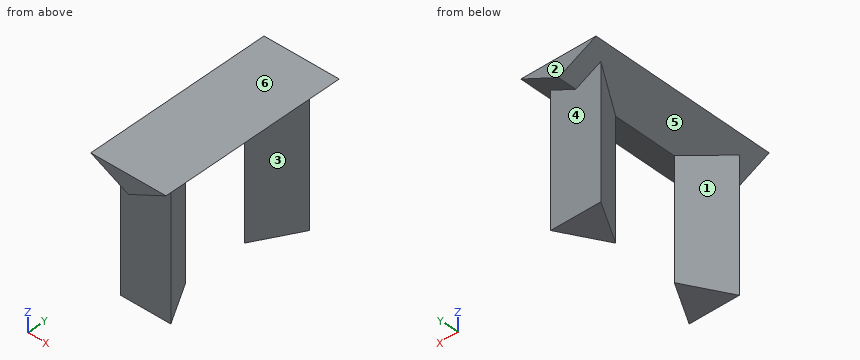
from build123d import *

# Parameters (mm, degrees)
F1_DEPTH = 150
F4_DEPTH = 110


with BuildPart() as f1:
    # F0 (on Front) → F1 (new body)
    with BuildSketch(Plane.XZ):
        Polygon((60, 0), (0, 0), (30, -15), align=None)
    extrude(amount=F1_DEPTH)

    # F3 (on offset) → F4 (join)
    with BuildSketch(Plane.XY.offset(-110)):
        Polygon((30, -100.3589838486), (10, -135), (50, -135), align=None)
        Polygon((30, -49.6410161514), (50, -15), (10, -15), align=None)
    extrude(amount=F4_DEPTH)


solid = f1.part
Can you work these out from the model? Positions are in its coordinate system, mm. Face numbers are marked on the shaded views. A direction names the side the tool comes from. Give positions to 0.01 mm unless a question says otherwise; leave off trailing zeros. Write each loop counter-clockwise with the first axis right and the second up, starting at its lowest first coordinate (ties: lowest second). Pieces come first, ordered by that corner, then holes. Notation, with made-up numbers: (36.25, 51.25) -> (64.25, 51.25) arc R27 ccw to (64.25, 76.25) -> close; hole circle Ø3 at (-35.5, 5.5). An arc over 180 degrees is marked (long way). Answer as a JSON object with one key per item and string values. Group by question number.
Item 1: I'm going to push flat-ended pins straight in: P1, Ø20, axis at x = 34.5, z = -35, coming from the -Y side; P2, Ø4, axis at x = 17, y = -106.5, coming from the -Z side; P3, Ø1, axis at x = 44, z = -73.5, coming from the +Y side. Where does each tip first touch, or does it pass through?
Item 2: Suppose I cut it at D-D (x = 46). Please give me the cut outline in (y, z).
Item 3: Please list where these lines run through material, in increasing order: line 1 (Y direction, x = 18, z = -18.5); line 2 (Y direction, x = 20, z = -44); line 3 (Z direction, x = 39, y = -79.5). Write a range as [from, to].
Item 4: Suppose I cut it at A-A (z = -95.5). Please give me the cut outline in (x, y).
Item 5: Suppose I cut it at C-C (y = -115). Please give me the cut outline in (x, z), plus the area to 3 significant figures.
Item 6: Suppose I cut it at B-B (x = 53). Please give me the cut outline in (y, z).
Item 7: For the marked faces 1, 2 and 3, which set-ups out of +Z, -Z, +X, -X, +Y, -Y let a thin tool reach every point of the face, with its end or its side?
Item 8: We'd pull the mould along Y, two halves only. Please class the marked faces 4, 5 and 6: +Y half, -Y half, draft (parallel to the pull), parting line (faces both ways), or undercut.
Findings:
{
 "1": {"P1": "stops at y = -135", "P2": "stops at z = -9.5", "P3": "stops at y = -15"},
 "2": {"outline": "(-150, -7) -> (-135, -7) -> (-135, -110) -> (-128.07, -110) -> (-128.07, -7) -> (-21.93, -7) -> (-21.93, -110) -> (-15, -110) -> (-15, -7) -> (0, -7) -> (0, 0) -> (-150, 0) -> close"},
 "3": {"line 1": "y = [-135, -121.14], [-28.86, -15]", "line 2": "y = [-135, -117.68], [-32.32, -15]", "line 3": "z = [-10.5, 0]"},
 "4": {"outline": "(10, -135) -> (50, -135) -> (30, -100.36) -> close; (10, -15) -> (30, -49.64) -> (50, -15) -> close"},
 "5": {"outline": "(0, 0) -> (21.55, -10.77) -> (21.55, -110) -> (38.45, -110) -> (38.45, -10.77) -> (60, 0) -> close", "area": "2,090 mm²"},
 "6": {"outline": "(-150, -3.5) -> (0, -3.5) -> (0, 0) -> (-150, 0) -> close"},
 "7": {"face 1": "-Z, -X", "face 2": "+Z, -Z, +X, -X, +Y", "face 3": "-Z, +X"},
 "8": {"face 4": "+Y half", "face 5": "undercut", "face 6": "draft"}
}
